Work out the finished part from the listing and answer in its coordinate system (mm). A direction names the side the tool comes from. Coordinates: 2 decimals unless noted, no trailing zeros. Loops run counter-clockwise (first coordinate to the right, second up) from the corner with the lowest first, then second, coordinate; pieces in that order, holes last. Notation, with made-up numbers: (89.25, -21.75) -> (107.25, -21.75) arc R26 ccw to (107.25, 13.25) -> close; hole circle Ø6 at (56.25, 65.25). An arc over 180 degrees is marked (long way). One line per question, with ' | ' between items.
```python
from build123d import *

# Parameters (mm, degrees)
SKETCH2_R           = 10
BOSS_EXTRUDE1_DEPTH = 30
SKETCH3_W           = 20
SKETCH3_H           = 20
BOSS_EXTRUDE2_DEPTH = 40
SKETCH4_R           = 5
CUT_EXTRUDE1_DEPTH  = 10


with BuildPart() as part:
    # Sketch2 → Boss-Extrude1 (new body, symmetric)
    with BuildSketch(Plane.XY):
        Circle(SKETCH2_R)
    extrude(amount=BOSS_EXTRUDE1_DEPTH, both=True)

    # Sketch3 → Boss-Extrude2 (add)
    with BuildSketch(Plane(origin=(0, 0, 0), x_dir=(1, 0, 0), z_dir=(0, 1, 0))):
        Rectangle(SKETCH3_W, SKETCH3_H)
    extrude(amount=BOSS_EXTRUDE2_DEPTH)

    # Sketch4 → Cut-Extrude1 (cut)
    with BuildSketch(Plane(origin=(0, 40, 0), x_dir=(1, 0, 0), z_dir=(0, 1, 0))):
        Circle(SKETCH4_R)
    extrude(amount=-CUT_EXTRUDE1_DEPTH, mode=Mode.SUBTRACT)


solid = part.part
```
1) For faces 1 (the face through (-2.17, -9.76, 0.42)), 2 (the face through (0, 30, 0)), 3 (the face through (10, 20, 0)), determine the directions among +Z, -Z, +X, -X, +Y, -Y from which every point of the face is accessible in a straight line to the end or side of a thin tool.
Check values:
face 1: none | face 2: +Y | face 3: +Z, -Z, +X, +Y, -Y
2) Find section A-A (z = 0). Write down the section's boundary in (x, y), plus the area to 3 significant figures.
Check values:
outline: (-10, 0) arc R10 ccw to (10, 0) -> (10, 40) -> (5, 40) -> (5, 30) -> (-5, 30) -> (-5, 40) -> (-10, 40) -> close | area: 857 mm^2
3) Find section B-B (x = 0). Write down the section's boundary in (y, z), plus the area to 3 significant figures.
Check values:
outline: (-10, -30) -> (10, -30) -> (10, -10) -> (40, -10) -> (40, -5) -> (30, -5) -> (30, 5) -> (40, 5) -> (40, 10) -> (10, 10) -> (10, 30) -> (-10, 30) -> close | area: 1,700 mm^2
4) Find section D-D (x = 3.75). Write down the section's boundary in (y, z).
Check values:
outline: (-9.27, -30) -> (9.27, -30) -> (9.27, -10) -> (40, -10) -> (40, -3.31) -> (30, -3.31) -> (30, 3.31) -> (40, 3.31) -> (40, 10) -> (9.27, 10) -> (9.27, 30) -> (-9.27, 30) -> close
5) The mould has two halves that part along Z. Classify faces 4 (the face through (0, 0, 30)), 5 (the face through (-1.08, 35.07, 4.88)), 6 (the face through (0, 0, -30)): released by +Z, released by -Z, zero draft, split by the parting line, or undercut.
Check values:
face 4: released by +Z | face 5: undercut | face 6: released by -Z
6) Find the intervals of material crossed by line 1 along Z through (x, y) = (0, 32.5); line 2 along Z through (x, y) = (6.5, 13), in increasing order.
Check values:
line 1: z = -10 to -5, 5 to 10 | line 2: z = -10 to 10
7) Flat-ended cylindrical pins translate along their axes: pin 1 (5 mm diameter, centred on x = -3.5, z = 13.5, fed in from +Y); pin 2 (6 mm diameter, centred on x = -1.5, y = 13, fed in from +Z); pin 3 (4 mm diameter, centred on x = -7, z = 19, fed in from +Y). Find the tip coordinate at first contact, or state that the pin passes through.
Check values:
pin 1: stops at y = 9.95 | pin 2: stops at z = 10 | pin 3: stops at y = 8.66
8) Find section C-C (y = 21.5). Write down the section's boundary in (x, z).
Check values:
outline: (-10, -10) -> (10, -10) -> (10, 10) -> (-10, 10) -> close
